For this review, use the dimensioned drawing (mm, ordinates from the lowest corner) and the shaded views. A direction names the side the tool comes from. Give positions to 0.01 mm unless a question says otherwise; leave off trailing zeros. Order: outer loops, then holes, each group sorted by start corner. A loop starts at its lowest first (then second) coordinate and runs counter-clockwise, first axis right, second up. Notation, with made-up numbers: (46, -7.5) - (102, -7.5) arc R11 cw to (102, 0.5) - close; hole circle Ø5 at (-31.5, 66). An arc over 180 degrees is marked (long way). Use a Markdown table: item, result. Add a question column.
1) We need section A-A on y = 3.5. Write out the cut boundary in (x, z), then the cut area to 3 significant figures.
2) Mouldability with a two-part tool opening along X and no side actions: class the marked faces 6, 7, 8 and 9 as released by +X, released by -X, zero draft, split by the parting line, or undercut.
3) Clearance check with flat-ended pins moving along their axes: P1, Ø1, axis at y = 9.5, z = 1.5, coming from the -X side; P2, Ø2, axis at y = 9, z = 2.5, coming from the +X side (1 decimal); P3, Ø2, axis at y = 3.5, z = 1, coming from the +X side (1 decimal); P4, Ø4, axis at x = 5, y = 8.5, coming from the -Z side. State where each tip first meets the part, or that it passes through.
4) We need section C-C on x = 8.7. Write out the cut boundary in (y, z).
5) We need section D-D on x = 5.75. Write out the cut boundary in (y, z).
6) Wall thickness on L1, parallel to Y at x = 3.5, z = 3.5; L2, parallel to Y at x = 6.75, z = 4; L3, parallel to Z at x = 7, y = 5.5: over which ranges is each line inside the solid? List them lowest first.
7) Machinability: for the marked faces 1, 2, 3, 4 and 5, which of the approach directions +Z, -Z, +X, -X, +Y, -Y give a long, thin tool a straight path to every point of the face, cutting with its end or side? Answer none if there is none.
8) We need section B-B on z = 4.4. Give the number of separate pieces and of enclosed holes in the cut face.
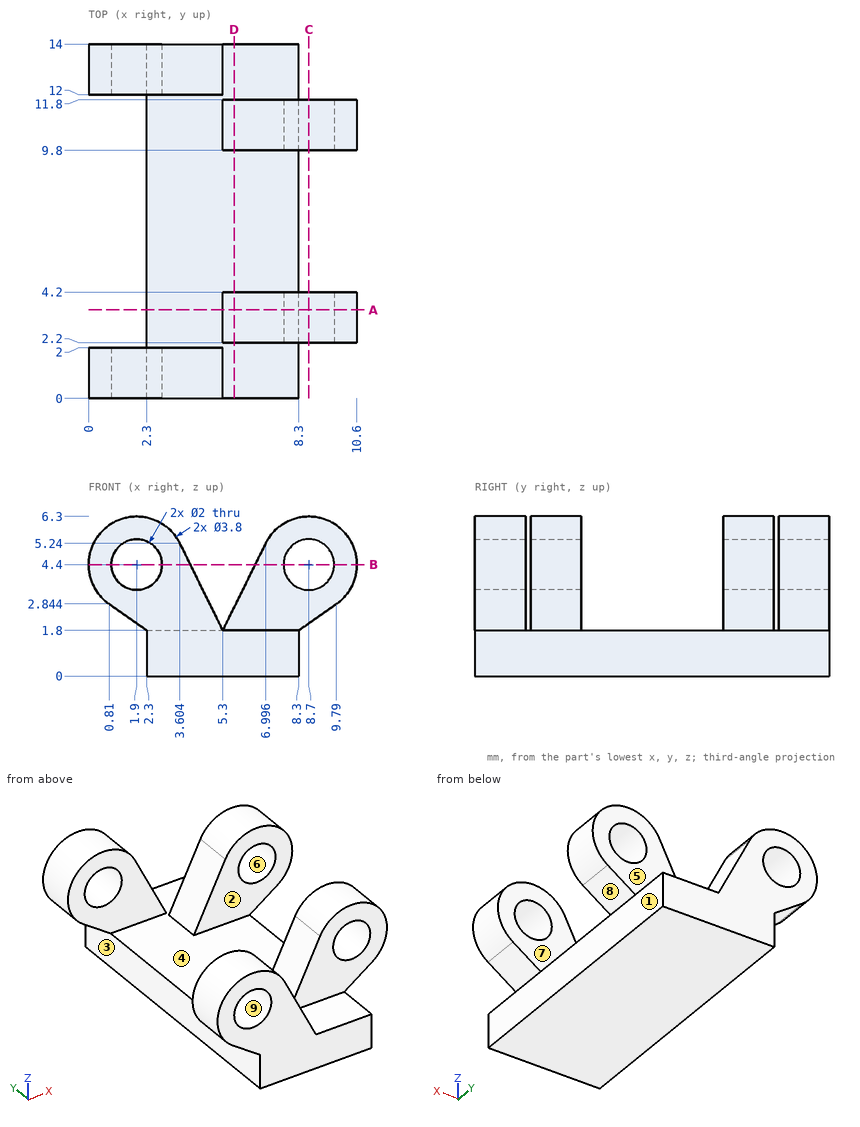
Checked values:
| question | item | result |
|---|---|---|
| 1 | outline | (2.3, 0) - (8.3, 0) - (8.3, 1.8) - (9.79, 2.84) arc R1.9 ccw (long way) to (7, 5.24) - (5.3, 1.8) - (2.3, 1.8) - close; hole circle Ø2 at (8.7, 4.4) |
| 1 | area | 23.5 mm² |
| 2 | face 6 | undercut |
| 2 | face 7 | zero draft |
| 2 | face 8 | released by +X |
| 2 | face 9 | undercut |
| 3 | P1 | x = 2.3 |
| 3 | P2 | x = 10.1 |
| 3 | P3 | x = 8.6 |
| 3 | P4 | z = 0 |
| 4 | outline | (2.2, 2.08) - (4.2, 2.08) - (4.2, 3.4) - (2.2, 3.4) - close; (2.2, 5.4) - (4.2, 5.4) - (4.2, 6.3) - (2.2, 6.3) - close; (9.8, 2.08) - (11.8, 2.08) - (11.8, 3.4) - (9.8, 3.4) - close; (9.8, 5.4) - (11.8, 5.4) - (11.8, 6.3) - (9.8, 6.3) - close |
| 5 | outline | (0, 0) - (14, 0) - (14, 1.8) - (11.8, 1.8) - (11.8, 2.71) - (9.8, 2.71) - (9.8, 1.8) - (4.2, 1.8) - (4.2, 2.71) - (2.2, 2.71) - (2.2, 1.8) - (0, 1.8) - close |
| 6 | L1 | 0 to 2, 12 to 14 |
| 6 | L2 | 2.2 to 4.2, 9.8 to 11.8 |
| 6 | L3 | 0 to 1.8 |
| 7 | face 1 | -Z, +X, +Y, -Y |
| 7 | face 2 | +Z, +X, -X |
| 7 | face 3 | -Z, -X, +Y, -Y |
| 7 | face 4 | +Z |
| 7 | face 5 | +Z, +X, -X, +Y |
| 8 | separate pieces | 8 |
| 8 | enclosed holes | 0 |
